from build123d import *

# Parameters (mm, degrees)
F0_W      = 57.525436
F0_H      = 68.329709
F1_DEPTH  = 25.4
F2_R      = 14.907727
F3_DEPTH  = 25.4
F4_W      = 49.749678
F4_H      = 3.633402
F5_DEPTH  = 25.4
F6_W      = 17.887524
F6_H      = 13.415642
F7_DEPTH  = 25.4
F8_W      = 31.582661
F8_H      = 6.428329
F8_W_2    = 31.023681
F8_H_2    = 6.42833
F9_DEPTH  = 25.4
F10_W     = 10.900209
F10_H     = 34.936577
F10_W_2   = 11.179707
F10_H_2   = 35.216067
F11_DEPTH = 25.4
F12_R     = 4.685148
F12_R_2   = 4.808572
F13_DEPTH = 25.4


with BuildPart() as f1:
    # F0 (on Top) → F1 (new body)
    with BuildSketch(Plane.XY):
        with Locations((1.752042, -4.234104)):
            Rectangle(F0_W, F0_H)
    extrude(amount=F1_DEPTH)

    # F2 (on Top) → F3 (join)
    with BuildSketch(Plane.XY):
        with Locations((3.003552, 36.584344)):
            Circle(F2_R)
    extrude(amount=F3_DEPTH)

    # F4 (on Top) → F5 (join)
    with BuildSketch(Plane.XY):
        with Locations((4.68051, 48.462778)):
            Rectangle(F4_W, F4_H)
    extrude(amount=F5_DEPTH)

    # F6 (on Top) → F7 (join)
    with BuildSketch(Plane.XY):
        with Locations((3.003553, 53.912882)):
            Rectangle(F6_W, F6_H)
    extrude(amount=F7_DEPTH)

    # F8 (on Top) → F9 (join)
    with BuildSketch(Plane.XY):
        with Locations((42.831245, 17.159609)):
            Rectangle(F8_W, F8_H)
        with Locations((-37.662617, 16.321131)):
            Rectangle(F8_W_2, F8_H_2)
    extrude(amount=F9_DEPTH)

    # F10 (on Top) → F11 (join)
    with BuildSketch(Plane.XY):
        with Locations((24.943721, -55.508465)):
            Rectangle(F10_W, F10_H)
        with Locations((-21.032811, -55.368719)):
            Rectangle(F10_W_2, F10_H_2)
    extrude(amount=F11_DEPTH)

    # F12 (on Top) → F13 (cut)
    with BuildSketch(Plane.XY):
        with Locations((11.388331, 38.820285)):
            Circle(F12_R)
        with Locations((-3.704268, 38.540792)):
            Circle(F12_R_2)
    extrude(amount=F13_DEPTH, mode=Mode.SUBTRACT)


solid = f1.part
Geometry check sheet. Reference: the model listing, model coordinates, mm. A direction names the side the tool comes from. Give positions to 0.01 mm unless a question says otherwise; leave off trailing zeros. Write each loop counter-clockwise with the first axis right and the second up, starting at its lowest first coordinate (ties: lowest second). Pieces come first, ordered by that corner, then holes. Notation, with made-up numbers: M -14,46 L 35,46 A18 ccw 35,76 Z; hole C -14,43.25 d10. An arc over 180 degrees is marked long. Answer as CSV lines item,"result". Start each with the question number.
Q1. Section check B-B, the plane y = -40.5. Record the cut outline in (x, z).
Q2. Section check C-C, the plane z = 18.75. Give the number of separate pieces and of enclosed holes in the cut face, then the cut area to 3 significant figures.
Q3. Material ranges on L1, parallel to Y at x = -20, z = 17; L2, parallel to X at y = 38, z = 11.5; L3, parallel to Y at x = -13.5, z = 18.5, recorded low to high.
Q4. Go/stop test with flat-tipped pins: pin 1 (11.5 mm diameter, centred on x = 21.5, z = 15, fed in from +Y); pin 2 (12.5 mm diameter, centred on y = -54.5, z = 14, fed in from +X); pin 3 (2 mm diameter, centred on x = -21.5, z = 10, fed in from +Y). Record where each tip stops, or that it passes through.
Q5. Section check A-A, the plane x = 28. Record the cut outline in (y, z).
Q6. Release check for a two-part mould opening along Y. For faces 4 (the face through (-14, 46.646, 13)), 5 (the face through (25, -72.977, 13)), 6 (the face through (30.394, -56, 13)) record: pulls with the +Y half, pulls with the -Y half, needs draft (parallel to the pull), parting line crosses it, or undercut.
Q7. Tool access check on faces 1 (the face through (21, 50.279, 13)), 2 (the face through (2, -38.399, 13)), 3 (the face through (-27.011, -13, 13)). Record the directions out of +Z, -Z, +X, -X, +Y, -Y that give a thin tool (end or side, any length) a straight path to the whole face; none if there is none.
Geometry says:
1,outline,"M -26.62,0 L -15.44,0 L -15.44,25.4 L -26.62,25.4 Z; M 19.49,0 L 30.39,0 L 30.39,25.4 L 19.49,25.4 Z"
2,separate pieces,"1"
2,enclosed holes,"2"
2,area,"5,730 mm^2"
3,L1,"-72.98 to 29.93, 46.65 to 50.28"
3,L2,"-11.84 to -8.48, 1.07 to 6.78, 16 to 17.84"
3,L3,"-38.4 to 29.93, 46.65 to 50.28"
4,pin 1,"y = 50.28"
4,pin 2,"x = 30.39"
4,pin 3,"y = 29.93"
5,outline,"M -72.98,0 L 29.93,0 L 29.93,25.4 L -72.98,25.4 Z; M 46.65,0 L 50.28,0 L 50.28,25.4 L 46.65,25.4 Z"
6,face 4,"undercut"
6,face 5,"pulls with the -Y half"
6,face 6,"needs draft"
7,face 1,"+Z, -Z, +X, +Y"
7,face 2,"+Z, -Z, -Y"
7,face 3,"+Z, -Z, -X, -Y"
